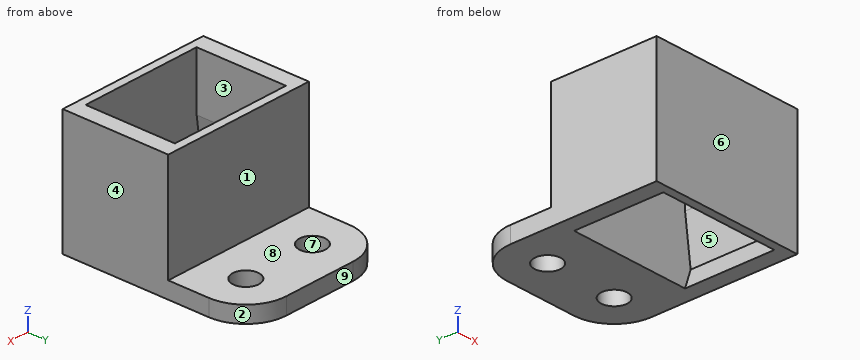
from build123d import *

# Parameters (mm, degrees)
SKETCH1_W           = 38
SKETCH1_H           = 26
SKETCH1_W_2         = 30
SKETCH1_H_2         = 22
BOSS_EXTRUDE1_DEPTH = 30
CUT_EXTRUDE1_DEPTH  = 22
SKETCH3_R           = 3.2
BOSS_EXTRUDE2_DEPTH = 4


with BuildPart() as part:
    # Sketch1 → Boss-Extrude1 (new body)
    with BuildSketch(Plane.XY):
        Rectangle(SKETCH1_W, SKETCH1_H)
        Rectangle(SKETCH1_W_2, SKETCH1_H_2, mode=Mode.SUBTRACT)
    extrude(amount=BOSS_EXTRUDE1_DEPTH)

    # Sketch2 → Cut-Extrude1 (cut)
    with BuildSketch(Plane.XZ.offset(-11)):
        Polygon((15, 0), (16.5, 4.5), (15, 16), align=None)
        Polygon((-15, 16), (-15, 0), (-16.5, 4.5), align=None)
    extrude(amount=CUT_EXTRUDE1_DEPTH, mode=Mode.SUBTRACT)

    # Sketch3 → Boss-Extrude2 (add)
    with BuildSketch(Plane(origin=(0, 0, 0), x_dir=(-1, 0, 0), z_dir=(0, 0, -1))):
        with BuildLine():
            Line((19, 13), (-19, 13))
            Line((-19, 13), (-19, 23))
            ThreePointArc((-19, 23), (-16.071067812, 30.071067812), (-9, 33))
            Line((-9, 33), (9, 33))
            ThreePointArc((9, 33), (16.071067812, 30.071067812), (19, 23))
            Line((19, 23), (19, 13))
        make_face()
        with Locations((-9, 23)):
            Circle(SKETCH3_R, mode=Mode.SUBTRACT)
        with Locations((9, 23)):
            Circle(SKETCH3_R, mode=Mode.SUBTRACT)
    extrude(amount=-BOSS_EXTRUDE2_DEPTH)


solid = part.part
For this review, take the finished solid that the model builds, in its own axes (mm). Face numbers are marked on the shaded views. A direction names the side the tool comes from. Give positions to 0.01 mm unless a question says otherwise; leave off trailing zeros. Order: outer loops, then holes, each group sorted by start corner. A loop starts at its lowest first (then second) coordinate and runs counter-clockwise, first axis right, second up. Notation, with made-up numbers: (37, -8) - (81, -8) arc R31 ccw to (81, 21) - close; hole circle Ø1 at (-37, -8.75). An arc over 180 degrees is marked (long way). Answer as a JSON object with one key per item and string values. Group by question number.
Item 1: Take a section at A-A on x = -2.5. Give the boundary of the cut face in (y, z).
Item 2: Take a section at B-B on y = -1. Give the boundary of the cut face in (x, z), and give its area (3 significant figures).
Item 3: Draft analysis for pull direction Y (two halves, no side actions). For the marked faces 6, 7, 8 and 9, state which applies: pulls with the +Y half, pulls with the -Y half, needs draft (parallel to the pull), parting line crosses it, or undercut.
Item 4: Take a section at C-C on z = 18. Give the boundary of the cut face in (x, y), and give its area (3 significant figures).
Item 5: Machinability: for the marked faces 1, 2, 3, 4 and 5, which of the approach directions +Z, -Z, +X, -X, +Y, -Y give a long, thin tool a straight path to every point of the face, cutting with its end or side? Answer none if there is none.
Item 6: Clearance check with a flat-ended pin moving along its axis: pin 1 Ø6 at (x, y) = (2.5, 18.5) entering from +Z. State where the tip first meets the part, or that it passes through.
Item 7: Wall thickness on line 1 along Y through (x, z) = (-9, 2.7); line 2 along Y through (x, z) = (-11.5, 28.25); line 3 along X through (y, z) = (-9.5, 16.5): over which ranges is each line inside the solid? List them lowest first.
Item 8: Take a section at D-D on y = 20.5. Give the boundary of the cut face in (x, z), and give its area (3 significant figures).
Reported:
{
 "1": {"outline": "(-13, 0) - (-11, 0) - (-11, 30) - (-13, 30) - close; (11, 0) - (33, 0) - (33, 4) - (13, 4) - (13, 30) - (11, 30) - close"},
 "2": {"outline": "(-19, 0) - (-15, 0) - (-16.5, 4.5) - (-15, 16) - (-15, 30) - (-19, 30) - close; (15, 0) - (19, 0) - (19, 30) - (15, 30) - (15, 16) - (16.5, 4.5) - close", "area": "216 mm^2"},
 "3": {"face 6": "pulls with the -Y half", "face 7": "undercut", "face 8": "needs draft", "face 9": "pulls with the +Y half"},
 "4": {"outline": "(-19, -13) - (19, -13) - (19, 13) - (-19, 13) - close; hole (-15, -11) - (15, -11) - (15, 11) - (-15, 11) - close", "area": "328 mm^2"},
 "5": {"face 1": "+Z, +X, -X, +Y", "face 2": "+Z, -Z, +X, +Y", "face 3": "+Z, -Z", "face 4": "+Z, -Z, +X, +Y, -Y", "face 5": "none"},
 "6": {"pin 1": "z = 4"},
 "7": {"line 1": "-13 to -11, 11 to 19.8, 26.2 to 33", "line 2": "-13 to -11, 11 to 13", "line 3": "-19 to -15, 15 to 19"},
 "8": {"outline": "(-19, 0) - (-11, 0) - (-11, 4) - (-19, 4) - close; (-7, 0) - (7, 0) - (7, 4) - (-7, 4) - close; (11, 0) - (19, 0) - (19, 4) - (11, 4) - close", "area": "120 mm^2"}
}
